Geometry check sheet. Reference: the model listing, model coordinates, mm. A direction names the side the tool comes from. Coordinates: 2 decimals unless noted, no trailing zeros. Write each loop counter-clockwise with the first axis right and the second up, starting at its lowest first coordinate (ties: lowest second). Pieces come first, ordered by that corner, then holes. Notation, with made-up numbers: (76.5, 55.5) -> (132.5, 55.5) arc R27 cw to (132.5, 92.5) -> close; hole circle Ø2 at (-33, 65.5). An arc over 180 degrees is marked (long way). One line per question, with ' | ' between items.
Autodesk Inventor part; units mm, degrees
ref_plane "YZ Plane" through (0, 0, 0) normal (1, 0, 0) x (0, 1, 0)
ref_plane "XZ Plane" through (0, 0, 0) normal (0, 1, 0) x (-1, 0, 0)
ref_plane "XY Plane" through (0, 0, 0) normal (0, 0, 1) x (1, 0, 0)
sketch "Esboço1" plane through (0, 0, 0) normal (0, 0, 1) x (1, 0, 0)
  line L0 (16, -12) -> (8, -12)
  line L1 (8, -12) -> (8, 4)
  line L2 (8, 4) -> (16, 4)
  line L3 (16, 4) -> (16, -12)
  point P0 (0, 0)
  dimension "d0" = 8
  dimension "d1" = 16
extrude "Extrusão1" add sketch "Esboço1" against normal blind 8
sketch "Esboço3" plane through (8, -12, 0) normal (-1, 0, 0) x (0, 0, 1)
  circle A0 centre (-3.6, 4) radius 2.4
  circle A1 centre (-3.6, 12) radius 2.4
  line L0 (0, 0) -> (-8, 0)
  line L1 (-3.6, 0) -> (-8, 0) construction
  line L2 (-8, 16) -> (-8, 0)
  line L3 (-8, 0) -> (-8, 4) construction
  spline S0 degree 2 poles (-3.6, 0) (-8, 0) (-8, 4) knots 1 1 1 2 2 2
  line L4 (0, 16) -> (-8, 16)
  line L5 (-3.6, 16) -> (-8, 16) construction
  line L6 (-8, 16) -> (-8, 12) construction
  spline S1 degree 2 poles (-3.6, 16) (-8, 16) (-8, 12) knots 1 1 1 2 2 2
  circle A2 centre (-3.6, 12) radius 2.5
  circle A3 centre (-3.6, 4) radius 2.5
  point P0 (0, 12)
  dimension "d14" = 5
  dimension "d15" = 5
extrude "Extrusão3" cut sketch "Esboço3" against normal blind 8 contours A0 | A1 | L2 L4 S1 | L0 L2 S0 | A2 | A3
sketch "Esboço4" plane through (8, -12, 0) normal (-1, 0, 0) x (0, 0, 1)
  circle A0 centre (-3.6, 12) radius 3.1
  circle A1 centre (-3.6, 4) radius 3.1
  point P0 (0, 12)
extrude "Extrusão4" cut sketch "Esboço4" against normal blind 1
sketch "Esboço5" plane through (16, -12, 0) normal (1, 0, 0) x (0, 0, -1)
  circle A0 centre (3.6, 12) radius 3.1
  circle A1 centre (3.6, 4) radius 3.1
  point P0 (0, 12)
extrude "Extrusão5" cut sketch "Esboço5" against normal blind 1
properties part number "_3DPrint"
(1) Material ranges on line 1 (Y direction, x = 15.3, z = -3.6); line 2 (Y direction, x = 13.75, z = -3.75); line 3 (Z direction, x = 10.75, y = -9), recorded low to high.
Answers below:
line 1: y = -12 to -11.1, -4.9 to -3.1, 3.1 to 4 | line 2: y = -12 to -10.5, -5.5 to -2.5, 2.5 to 4 | line 3: z = -7.92 to -5.89, -1.31 to 0
(2) Draft check along Y on faces 4 (the face through (8, -4, -4)), 5 (the face through (8.493, 0.931, -0.643)), 6 (the face through (12, 4, -2)). Enter one of: pulls with the +Y half, pulls with the -Y half, needs draft (parallel to the pull), parting line crosses it, or undercut.
Answers below:
face 4: needs draft | face 5: undercut | face 6: pulls with the +Y half
(3) Cross-section at B-B (x = 14.5). Count the separate pieces of the cut face and the enclosed holes in it, plus the area to 3 significant figures.
Answers below:
separate pieces: 1 | enclosed holes: 2 | area: 82.9 mm²
(4) Tool access check on faces 1 (the face through (15.507, 0.931, -6.557)), 2 (the face through (12, -12, -2)), 3 (the face through (8.493, -7.069, -0.643)). Record the directions out of +Z, -Z, +X, -X, +Y, -Y that give a thin tool (end or side, any length) a straight path to the whole face; none if there is none.
Answers below:
face 1: +X | face 2: +Z, -Z, +X, -X, -Y | face 3: -X
(5) Cross-section at A-A (z = -2.5). Record the cut outline in (x, y) (3 decimals).
Answers below:
outline: (8, -12) -> (16, -12) -> (16, -10.898) -> (15, -10.898) -> (15, -10.245) -> (9, -10.245) -> (9, -10.898) -> (8, -10.898) -> close; (8, -5.102) -> (9, -5.102) -> (9, -5.755) -> (15, -5.755) -> (15, -5.102) -> (16, -5.102) -> (16, -2.898) -> (15, -2.898) -> (15, -2.245) -> (9, -2.245) -> (9, -2.898) -> (8, -2.898) -> close; (8, 2.898) -> (9, 2.898) -> (9, 2.245) -> (15, 2.245) -> (15, 2.898) -> (16, 2.898) -> (16, 4) -> (8, 4) -> close
(6) Depth check by flat-ended pin: P1, Ø1.9, axis at y = -7.5, z = -4, coming from the +X side (1 decimal). Enter the tip coordinate at first touch or a pass-through.
Answers below:
P1: passes through
